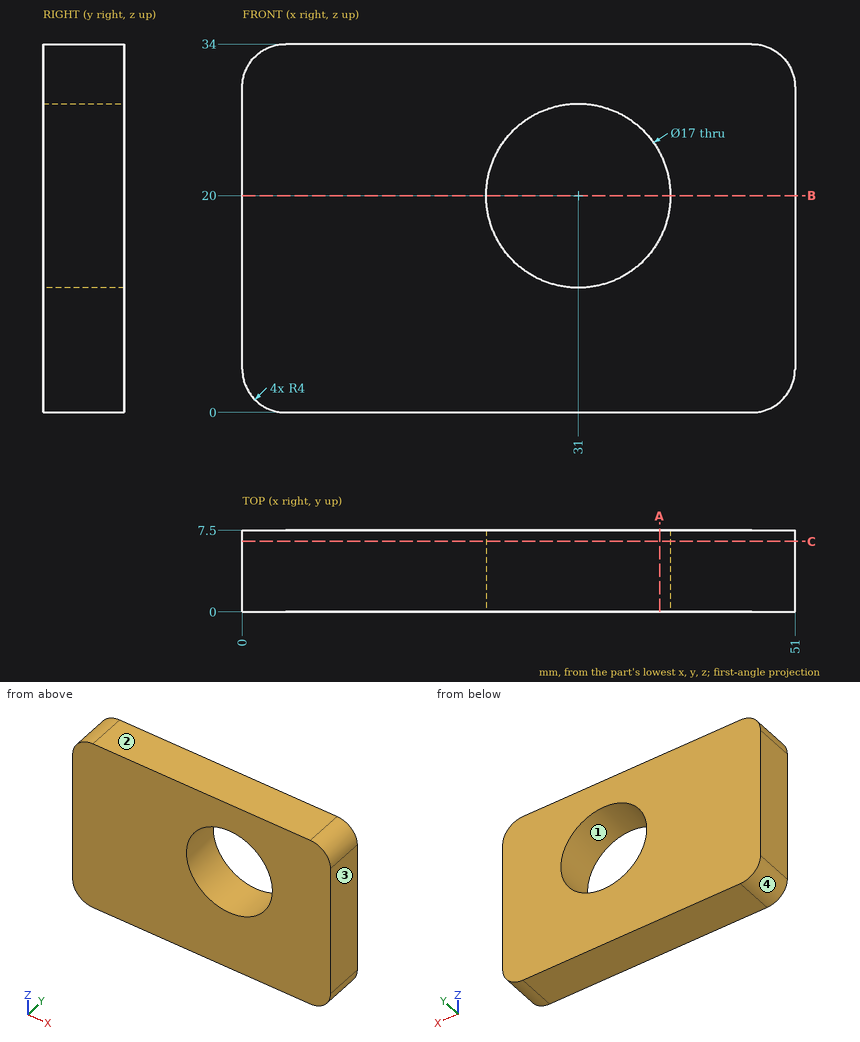
Geometry: see drawing. Coordinates: mm, zero at the bounding-box minimum. Coordinates: 2 decimals unless noted, no trailing zeros. Loops run counter-clockwise (first coordinate to the right, second up) from the corner with the lowest first, then second, coordinate; pieces in that order, holes last. Notation, with made-up numbers: (32.5, 20) - (58.5, 20) arc R14 ccw to (58.5, 27) - close; hole circle Ø1 at (39, 85). An arc over 180 degrees is marked (long way). Put each result on its own line as item: value. Start each with the question number.
Q1. Cut plane C-C, the plane y = 6.5. Return loops of the section in (x, z), and give its area (3 significant figures).
Q2. Cut plane B-B, the plane z = 20. Return loops of the section in (x, y), and give its area (3 significant figures).
Q3. Line query: line 1 (X direction, y = 5.25, z = 20); line 2 (X direction, y = 4.25, z = 25.5); line 3 (X direction, y = 6.5, z = 31). Output: solid intervals per line, ascending.
Q4. Pull-direction query (Z, two-part tool) for the marked faces 1, 2, 3 and 4; classes: released by +Z, released by -Z, zero draft, split by the parting line, or undercut.
Q5. Cut plane A-A, the plane x = 38.5. Return loops of the section in (y, z), and give its area (3 significant figures).
Filled sheet:
1. outline: (0, 4) arc R4 ccw to (4, 0) - (47, 0) arc R4 ccw to (51, 4) - (51, 30) arc R4 ccw to (47, 34) - (4, 34) arc R4 ccw to (0, 30) - close; hole circle Ø17 at (31, 20)
1. area: 1,490 mm²
2. outline: (0, 0) - (22.5, 0) - (22.5, 7.5) - (0, 7.5) - close; (39.5, 0) - (51, 0) - (51, 7.5) - (39.5, 7.5) - close
2. area: 255 mm²
3. line 1: 0 to 22.5, 39.5 to 51
3. line 2: 0 to 24.52, 37.48 to 51
3. line 3: 0.13 to 50.87
4. face 1: undercut
4. face 2: released by +Z
4. face 3: zero draft
4. face 4: released by -Z
5. outline: (0, 0) - (7.5, 0) - (7.5, 16) - (0, 16) - close; (0, 24) - (7.5, 24) - (7.5, 34) - (0, 34) - close
5. area: 195 mm²
